Geometry check sheet. Reference: the model listing, model coordinates, mm. Face numbers are marked on the shaded views. Coordinates: 2 decimals unless noted, no trailing zeros. Write each loop counter-clockwise with the first axis right and the second up, starting at its lowest first coordinate (ties: lowest second). Pieces come first, ordered by that corner, then holes. Notation, with made-up numbers: M -11.75,28.25 L 12.25,28.25 A14 cw 12.25,39.25 Z; hole C 19.25,16 d11. An arc over 180 degrees is marked long. Put each result on its own line as item: value. Start each with the question number.
1) Mould release check, pull along X, two halves, no side actions. Record for the marked faces 1, 2 and 3: released by +X, released by -X, zero draft, split by the parting line, or undercut.
2) Cross-section at A-A on x = -40. Record the cut outline in (y, z).
3) Cross-section at D-D on y = -30. Record the cut outline in (x, z).
4) Cross-section at C-C on x = 45. Record the cut outline in (y, z).
5) Scan lines: line 1 along Y through (x, z) = (-96.25, 4); line 2 along Y through (x, z) = (50, 2.25); line 3 along X through (y, z) = (-34, 2.5). Record each from-to range of solid material in increasing order.
6) Cross-section at B-B on z = 8.5. Record the cut outline in (x, y).
7) Gauge pin test, flat ends, axial feed: pin 1 (1 mm diameter, centred on x = 55.5, y = 36, fed in from -Z); pin 2 (5.5 mm diameter, centred on x = -91.11, y = -43.5, fed in from +Z); pin 3 (4 mm diameter, centred on x = 66.66, y = 41.03, fed in from +Z); pin 4 (4.5 mm diameter, centred on x = -31, y = 45.5, fed in from -Z). Record the tip position at first contact, or that the pin passes through.
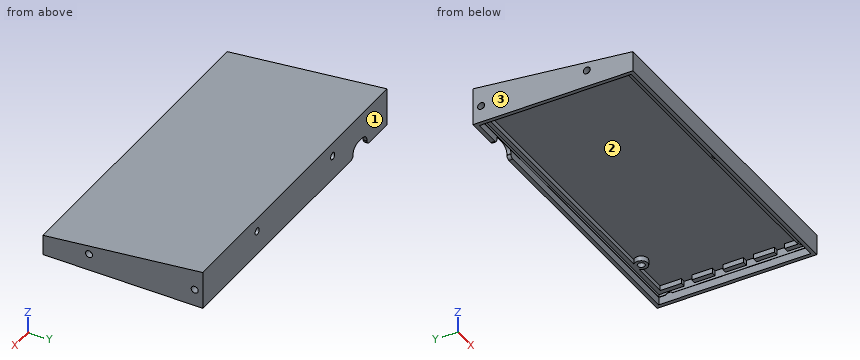
from build123d import *

# Parameters (mm, degrees)
SKETCH1_R           = 2.15
SKETCH1_W           = 3
SKETCH1_H           = 12.65
SKETCH1_H_2         = 12.75
BOSS_EXTRUDE1_DEPTH = 3.15085709
BOSS_EXTRUDE2_START = 3.150857
SKETCH1_3_R         = 2.15
SKETCH1_3_W         = 3
SKETCH1_3_H         = 6.4
SKETCH1_3_H_2       = 12.65
SKETCH1_3_H_3       = 12.75
SKETCH1_3_H_4       = 6.3
BOSS_EXTRUDE2_DEPTH = 3
SKETCH1_4_W         = 194.976
SKETCH1_4_H         = 98.329
SKETCH1_4_W_2       = 189.776
SKETCH1_4_H_2       = 93.129
BOSS_EXTRUDE4_DEPTH = 6.15085709
BOSS_EXTRUDE5_DEPTH = 194.976
SKETCH5_R           = 2.15
CUT_EXTRUDE2_DEPTH  = 4
SKETCH6_R           = 2.15
CUT_EXTRUDE3_DEPTH  = 4
CUT_EXTRUDE4_START  = -190.976
SKETCH6_2_R         = 2.15
CUT_EXTRUDE4_DEPTH  = 4
BOSS_EXTRUDE6_START = -1.6
SKETCH1_5_W         = 194.976
SKETCH1_5_H         = 98.329
SKETCH1_5_W_2       = 189.776
SKETCH1_5_H_2       = 93.129
BOSS_EXTRUDE6_DEPTH = 1.6
SKETCH7_R           = 3
CUT_EXTRUDE5_DEPTH  = 2.6
CUT_EXTRUDE6_START  = -194.976
SKETCH7_2_R         = 3
CUT_EXTRUDE6_DEPTH  = 2.6
BOSS_EXTRUDE7_START = -1
SKETCH9_W           = 2.4
SKETCH9_H           = 87.377932023
SKETCH9_H_2         = 4.078932023
SKETCH9_W_2         = 190.176
SKETCH9_H_3         = 2.4
SKETCH9_H_4         = 4.472135954
BOSS_EXTRUDE7_DEPTH = 5.8
CUT_EXTRUDE7_DEPTH  = 2.4
FILLET1_R           = 2


with BuildPart() as part:
    # Sketch1 → Boss-Extrude1 (new body)
    # profile 1 of 5: a face of its own
    with BuildSketch(Plane.XY):
        Polygon((94.888, 46.5645), (-94.888, 46.5645), (-94.888, -46.5645), (94.888, -46.5645), (94.888, -32.548850543), (91.888, -32.548850543), (91.888, -40.5645), (-87.888, -40.5645), (-87.888, 44.0645), (64.046820121, 44.0645), (69.267179879, 44.0645), (91.888, 44.0645), (91.888, 31.001149457), (94.888, 31.001149457), align=None)
        with Locations(Location((-91.11, -43.4975, 0), (0, 0, 180))):
            Circle(SKETCH1_R, mode=Mode.SUBTRACT)
        with Locations(Location((0.203, -43.4975, 0), (0, 0, 180))):
            Circle(SKETCH1_R, mode=Mode.SUBTRACT)
        with Locations(Location((91.389, -43.4975, 0), (0, 0, 180))):
            Circle(SKETCH1_R, mode=Mode.SUBTRACT)
        with Locations(Location((-91.11, 26.5025, 0), (0, 0, 180))):
            Circle(SKETCH1_R, mode=Mode.SUBTRACT)
    # profile 2 of 5: a face of its own
    with BuildSketch(Plane.XY):
        with Locations((93.388, 18.276149457)):
            Rectangle(SKETCH1_W, SKETCH1_H)
    # profile 3 of 5: a face of its own
    with BuildSketch(Plane.XY):
        with Locations((93.388, -0.823850543)):
            Rectangle(SKETCH1_W, SKETCH1_H_2)
    # profile 4 of 5: a face of its own
    with BuildSketch(Plane.XY):
        with Locations((93.388, -19.823850543)):
            Rectangle(SKETCH1_W, SKETCH1_H)
    # profile 5 of 5: a face of its own
    with BuildSketch(Plane.XY):
        with BuildLine():
            ThreePointArc((64.046820121, 44.0645), (66.657, 37.0335), (69.267179879, 44.0645))
            Line((69.267179879, 44.0645), (64.046820121, 44.0645))
        make_face()
        with Locations(Location((66.657, 41.0335, 0), (0, 0, 180))):
            Circle(SKETCH1_R, mode=Mode.SUBTRACT)
    extrude(amount=BOSS_EXTRUDE1_DEPTH)

    # Sketch1<3> → Boss-Extrude2 (add)
    # profile 1 of 15: a face of its own
    with BuildSketch(Plane.XY.offset(BOSS_EXTRUDE2_START)):
        Polygon((94.888, 46.5645), (-94.888, 46.5645), (-94.888, -46.5645), (94.888, -46.5645), (94.888, -32.548850543), (91.888, -32.548850543), (91.888, -40.5645), (-87.888, -40.5645), (-87.888, 44.0645), (64.046820121, 44.0645), (69.267179879, 44.0645), (91.888, 44.0645), (91.888, 31.001149457), (94.888, 31.001149457), align=None)
        with Locations(Location((-91.11, -43.4975, 0), (0, 0, 180))):
            Circle(SKETCH1_3_R, mode=Mode.SUBTRACT)
        with Locations(Location((0.203, -43.4975, 0), (0, 0, 180))):
            Circle(SKETCH1_3_R, mode=Mode.SUBTRACT)
        with Locations(Location((91.389, -43.4975, 0), (0, 0, 180))):
            Circle(SKETCH1_3_R, mode=Mode.SUBTRACT)
        with Locations(Location((-91.11, 26.5025, 0), (0, 0, 180))):
            Circle(SKETCH1_3_R, mode=Mode.SUBTRACT)
    # profile 2 of 15: a face of its own
    with BuildSketch(Plane.XY.offset(BOSS_EXTRUDE2_START)):
        with Locations((93.388, 8.751149457)):
            Rectangle(SKETCH1_3_W, SKETCH1_3_H)
    # profile 3 of 15: a face of its own
    with BuildSketch(Plane.XY.offset(BOSS_EXTRUDE2_START)):
        with Locations((93.388, 18.276149457)):
            Rectangle(SKETCH1_3_W, SKETCH1_3_H_2)
    # profile 4 of 15: a face of its own
    with BuildSketch(Plane.XY.offset(BOSS_EXTRUDE2_START)):
        with BuildLine():
            Line((91.888, 24.601149457), (91.888, 31.001149457))
            Line((91.888, 31.001149457), (91.888, 44.0645))
            Line((91.888, 44.0645), (69.267179879, 44.0645))
            ThreePointArc((69.267179879, 44.0645), (66.657, 37.0335), (64.046820121, 44.0645))
            Line((64.046820121, 44.0645), (-87.888, 44.0645))
            Line((-87.888, 44.0645), (-87.888, -40.5645))
            Line((-87.888, -40.5645), (91.888, -40.5645))
            Line((91.888, -40.5645), (91.888, -32.548850543))
            Line((91.888, -32.548850543), (91.888, -26.148850543))
            Line((91.888, -26.148850543), (91.888, -13.498850543))
            Line((91.888, -13.498850543), (91.888, -7.198850543))
            Line((91.888, -7.198850543), (91.888, 5.551149457))
            Line((91.888, 5.551149457), (91.888, 11.951149457))
            Line((91.888, 11.951149457), (91.888, 24.601149457))
        make_face()
    # profile 5 of 15: a face of its own
    with BuildSketch(Plane.XY.offset(BOSS_EXTRUDE2_START)):
        with Locations((93.388, -0.823850543)):
            Rectangle(SKETCH1_3_W, SKETCH1_3_H_3)
    # profile 6 of 15: a face of its own
    with BuildSketch(Plane.XY.offset(BOSS_EXTRUDE2_START)):
        with Locations((93.388, -10.348850543)):
            Rectangle(SKETCH1_3_W, SKETCH1_3_H_4)
    # profile 7 of 15: a face of its own
    with BuildSketch(Plane.XY.offset(BOSS_EXTRUDE2_START)):
        with Locations((93.388, -19.823850543)):
            Rectangle(SKETCH1_3_W, SKETCH1_3_H_2)
    # profile 8 of 15: a face of its own
    with BuildSketch(Plane.XY.offset(BOSS_EXTRUDE2_START)):
        with Locations((93.388, -29.348850543)):
            Rectangle(SKETCH1_3_W, SKETCH1_3_H)
    # profile 9 of 15: a face of its own
    with BuildSketch(Plane.XY.offset(BOSS_EXTRUDE2_START)):
        with Locations((93.388, 27.801149457)):
            Rectangle(SKETCH1_3_W, SKETCH1_3_H)
    # profile 10 of 15: a face of its own
    with BuildSketch(Plane.XY.offset(BOSS_EXTRUDE2_START)):
        with BuildLine():
            ThreePointArc((64.046820121, 44.0645), (66.657, 37.0335), (69.267179879, 44.0645))
            Line((69.267179879, 44.0645), (64.046820121, 44.0645))
        make_face()
        with Locations(Location((66.657, 41.0335, 0), (0, 0, 180))):
            Circle(SKETCH1_3_R, mode=Mode.SUBTRACT)
    # profile 11 of 15: a face of its own
    with BuildSketch(Plane.XY.offset(BOSS_EXTRUDE2_START)):
        with Locations(Location((66.657, 41.0335, 0), (0, 0, 180))):
            Circle(SKETCH1_3_R)
    # profile 12 of 15: a face of its own
    with BuildSketch(Plane.XY.offset(BOSS_EXTRUDE2_START)):
        with Locations(Location((91.389, -43.4975, 0), (0, 0, 180))):
            Circle(SKETCH1_3_R)
    # profile 13 of 15: a face of its own
    with BuildSketch(Plane.XY.offset(BOSS_EXTRUDE2_START)):
        with Locations(Location((0.203, -43.4975, 0), (0, 0, 180))):
            Circle(SKETCH1_3_R)
    # profile 14 of 15: a face of its own
    with BuildSketch(Plane.XY.offset(BOSS_EXTRUDE2_START)):
        with Locations(Location((-91.11, -43.4975, 0), (0, 0, 180))):
            Circle(SKETCH1_3_R)
    # profile 15 of 15: a face of its own
    with BuildSketch(Plane.XY.offset(BOSS_EXTRUDE2_START)):
        with Locations(Location((-91.11, 26.5025, 0), (0, 0, 180))):
            Circle(SKETCH1_3_R)
    extrude(amount=BOSS_EXTRUDE2_DEPTH)

    # Sketch1<4> → Boss-Extrude4 (add)
    with BuildSketch(Plane.XY):
        Rectangle(SKETCH1_4_W, SKETCH1_4_H)
        Rectangle(SKETCH1_4_W_2, SKETCH1_4_H_2, mode=Mode.SUBTRACT)
    extrude(amount=BOSS_EXTRUDE4_DEPTH)

    # Sketch4 → Boss-Extrude5 (add)
    with BuildSketch(Plane.ZY.offset(97.488)):
        Polygon((6.15085709, 49.1645), (17, 49.1645), (6.15085709, -49.1645), align=None)
    extrude(amount=-BOSS_EXTRUDE5_DEPTH)

    # Sketch5 → Cut-Extrude2 (cut)
    with BuildSketch(Plane(origin=(0, 49.1645, 0), x_dir=(1, 0, 0), z_dir=(0, 1, 0))):
        with Locations(Location((-40, -8.5, 0), (0, 0, 270))):
            Circle(SKETCH5_R)
        with Locations(Location((40, -8.5, 0), (0, 0, 270))):
            Circle(SKETCH5_R)
    extrude(amount=-CUT_EXTRUDE2_DEPTH, mode=Mode.SUBTRACT)

    # Sketch6 → Cut-Extrude3 (cut)
    with BuildSketch(Plane(origin=(97.488, 0, 0), x_dir=(0, 0, -1), z_dir=(1, 0, 0))):
        with Locations((-4, 44.1645)):
            Circle(SKETCH6_R)
        with Locations((-4, -20.8355)):
            Circle(SKETCH6_R)
    extrude(amount=-CUT_EXTRUDE3_DEPTH, mode=Mode.SUBTRACT)

    # Sketch6<2> → Cut-Extrude4 (cut)
    with BuildSketch(Plane(origin=(97.488, 0, 0), x_dir=(0, 0, -1), z_dir=(1, 0, 0)).offset(CUT_EXTRUDE4_START)):
        with Locations((-4, 44.1645)):
            Circle(SKETCH6_2_R)
        with Locations((-4, -20.8355)):
            Circle(SKETCH6_2_R)
    extrude(amount=-CUT_EXTRUDE4_DEPTH, mode=Mode.SUBTRACT)

    # Sketch1<5> → Boss-Extrude6 (add)
    with BuildSketch(Plane.XY.offset(BOSS_EXTRUDE6_START)):
        Rectangle(SKETCH1_5_W, SKETCH1_5_H)
        Rectangle(SKETCH1_5_W_2, SKETCH1_5_H_2, mode=Mode.SUBTRACT)
    extrude(amount=BOSS_EXTRUDE6_DEPTH)

    # Sketch7 → Cut-Extrude5 (cut)
    with BuildSketch(Plane.ZY.offset(97.488)):
        with Locations((-3.6, 40.4495)):
            Circle(SKETCH7_R)
    extrude(amount=-CUT_EXTRUDE5_DEPTH, mode=Mode.SUBTRACT)

    # Sketch7<2> → Cut-Extrude6 (cut)
    with BuildSketch(Plane.ZY.offset(97.488).offset(CUT_EXTRUDE6_START)):
        with Locations((-3.6, 40.4495)):
            Circle(SKETCH7_2_R)
    extrude(amount=CUT_EXTRUDE6_DEPTH, mode=Mode.SUBTRACT)

    # Sketch9 → Boss-Extrude7 (add)
    with BuildSketch(Plane(origin=(0, 0, -1.6), x_dir=(-1, 0, 0), z_dir=(0, 0, -1)).offset(BOSS_EXTRUDE7_START)):
        Polygon((-97.488, 49.1645), (-97.488, 42.685567977), (-95.088, 42.685567977), (-95.088, 46.7645), (-95.088, 49.1645), align=None)
        Polygon((-95.088, 49.1645), (-95.088, 46.7645), (95.088, 46.7645), (97.488, 46.7645), (97.488, 49.1645), align=None)
        with Locations((-96.288, -5.475533989)):
            Rectangle(SKETCH9_W, SKETCH9_H)
        with Locations((96.288, 44.725033989)):
            Rectangle(SKETCH9_W, SKETCH9_H_2)
        with Locations((96.288, -5.475533989)):
            Rectangle(SKETCH9_W, SKETCH9_H)
        with Locations((0, -47.9645)):
            Rectangle(SKETCH9_W_2, SKETCH9_H_3)
        with Locations((-96.288, 40.4495)):
            Rectangle(SKETCH9_W, SKETCH9_H_4)
        with Locations((96.288, 40.4495)):
            Rectangle(SKETCH9_W, SKETCH9_H_4)
    extrude(amount=BOSS_EXTRUDE7_DEPTH)

    # Sketch10 → Cut-Extrude7 (cut)
    with BuildSketch(Plane(origin=(0, 49.1645, 0), x_dir=(1, 0, 0), z_dir=(0, 1, 0))):
        with BuildLine():
            Line((-66.44559, 9.005), (-71.48559, 9.005))
            ThreePointArc((-71.48559, 9.005), (-74.024758171, 8.304132264), (-75.844887535, 6.4))
            Line((-75.844887535, 6.4), (-76.43559, 6.4))
            Line((-76.43559, 6.4), (-76.43559, 4.055))
            ThreePointArc((-76.43559, 4.055), (-74.985768567, 0.554821433), (-71.48559, -0.895))
            Line((-71.48559, -0.895), (-66.44559, -0.895))
            ThreePointArc((-66.44559, -0.895), (-62.945411433, 0.554821433), (-61.49559, 4.055))
            Line((-61.49559, 4.055), (-61.49559, 6.4))
            Line((-61.49559, 6.4), (-62.086292465, 6.4))
            ThreePointArc((-62.086292465, 6.4), (-63.906421829, 8.304132264), (-66.44559, 9.005))
        make_face()
    extrude(amount=-CUT_EXTRUDE7_DEPTH, mode=Mode.SUBTRACT)

    # Fillet1
    fillet1_edges = [part.edges().sort_by_distance(p)[0] for p in [
        (-76.43559, 47.9645, -6.4),
        (-61.49559, 47.9645, -6.4),
    ]]
    fillet(fillet1_edges, radius=FILLET1_R)


solid = part.part
Answer key:
1. face 1: zero draft
1. face 2: undercut
1. face 3: released by -X
2. outline: M -49.16,-6.4 L -46.76,-6.4 L -46.76,-1.6 L -46.56,-1.6 L -46.56,0 L -40.56,0 L -40.56,3.15 L 44.06,3.15 L 44.06,0 L 46.56,0 L 46.56,-1.6 L 46.76,-1.6 L 46.76,-6.4 L 49.16,-6.4 L 49.16,6.35 L 45.16,6.35 L 45.16,10.65 L 49.16,10.65 L 49.16,17 L -49.16,6.15 Z
3. outline: M -97.49,-6.4 L -95.09,-6.4 L -95.09,-1.6 L -94.89,-1.6 L -94.89,0 L -87.89,0 L -87.89,3.15 L 94.89,3.15 L 94.89,-1.6 L 95.09,-1.6 L 95.09,-6.4 L 97.49,-6.4 L 97.49,8.27 L -97.49,8.27 Z
4. outline: M -49.16,-6.4 L -46.76,-6.4 L -46.76,-1.6 L -46.56,-1.6 L -46.56,0 L -40.56,0 L -40.56,3.15 L 44.06,3.15 L 44.06,0 L 46.56,0 L 46.56,-1.6 L 46.76,-1.6 L 46.76,-6.4 L 49.16,-6.4 L 49.16,17 L -49.16,6.15 Z
5. line 1: y = -49.16 to -22.99, -18.69 to 42.01, 46.31 to 49.16
5. line 2: y = -49.16 to -40.56, 44.06 to 49.16
5. line 3: x = -97.49 to -87.89, 91.89 to 97.49
6. outline: M -97.49,-27.87 L 97.49,-27.87 L 97.49,49.16 L 42.15,49.16 L 42.15,45.16 L 37.85,45.16 L 37.85,49.16 L -37.85,49.16 L -37.85,45.16 L -42.15,45.16 L -42.15,49.16 L -97.49,49.16 Z
7. pin 1: stops at z = 3.15
7. pin 2: stops at z = 7.08
7. pin 3: stops at z = 16.32
7. pin 4: stops at z = -6.4
